Autodesk Inventor part; units mm, degrees
ref_plane "YZ Plane" through (0, 0, 0) normal (1, 0, 0) x (0, 1, 0)
ref_plane "XZ Plane" through (0, 0, 0) normal (0, 1, 0) x (-1, 0, 0)
ref_plane "XY Plane" through (0, 0, 0) normal (0, 0, 1) x (1, 0, 0)
sketch "Skizze1" plane through (0, 0, 0) normal (0, 1, 0) x (-1, 0, 0)
  circle A0 centre (0, 0) radius 45
  circle A1 centre (0, 0) radius 47.5
  dimension "d0" = 90
  dimension "d1" = 95
extrude "Extrusion1" add sketch "Skizze1" along normal blind 10
sketch "Skizze2" plane through (0, 0, 0) normal (0, -1, 0) x (1, 0, 0)
  circle A0 centre (0, 0) radius 41.5
  circle A1 centre (0, 0) radius 50
  dimension "d4" = 83
  dimension "d5" = 100
extrude "Extrusion2" add sketch "Skizze2" along normal blind 3
sketch "Skizze3" plane through (0, -3, 0) normal (0, -1, 0) x (1, 0, 0)
  circle A0 centre (0, 0) radius 41.5
  circle A1 centre (0, 0) radius 44
  dimension "d8" = 83
  dimension "d9" = 88
extrude "Extrusion3" add sketch "Skizze3" along normal blind 5
sketch "Skizze4" plane through (0, 0, 0) normal (0, 1, 0) x (1, 0, 0)
  line L0 (-86, 0) -> (65, 0) construction
  line L1 (-86, 15) -> (65, 15)
  line L2 (-86, -15) -> (65, -15)
  line L3 (-86, 15) -> (-86, -15)
  line L4 (65, -15) -> (65, 15)
  point P0 (0, 0)
  dimension "d12" = 15
  dimension "d13" = 15
extrude "Extrusion4" cut sketch "Skizze4" along normal up to surface (10 mm away)
sketch "Skizze5" plane through (0, 10, 0) normal (0, 1, 0) x (1, 0, 0)
  line L0 (0, 0) -> (0, 69) construction
  line L1 (-1.5, 0) -> (-1.5, 46.3972)
  line L2 (1.5, 0) -> (1.5, 46.3972)
  line L3 (-1.5, 0) -> (1.5, 0)
  line L4 (-1.5, 46.3972) -> (1.5, 46.3972)
  dimension "d16" = 1.5
extrude "Extrusion5" cut sketch "Skizze5" against normal up to surface (10 mm away)
properties part number "Teesiebhalter"
For this review, take the finished solid that the model builds, in its own axes (mm). A direction names the side the tool comes from. Give positions to 0.01 mm unless a question says otherwise; leave off trailing zeros. Loops run counter-clockwise (first coordinate to the right, second up) from the corner with the lowest first, then second, coordinate; pieces in that order, holes last.
Item 1: Take a section at D-D, the plane z = 36.5. State the section outline as (x, y) points.
Item 2: Take a section at C-C, the plane x = 0. State the section outline as (y, z) points, and give its area (3 significant figures).
Item 3: Take a section at B-B, the plane y = 2.75. State the section outline as (x, z) points (3 decimals), and give its area (3 significant figures).
Item 4: Insertion check: pin 1 (8 mm diameter, centred on y = -3.5, z = -12.5, fed in from -X); pin 2 (8 mm diameter, centred on x = 25.5, z = 28.5, fed in from +Y); pin 3 (10 mm diameter, centred on x = 7, y = 2, fed in from +Z); pin 4 (10 mm diameter, centred on y = 6, z = 4, fed in from -X). Each pin has a flat end and moves straight along its axis. Give the tip position at first contact, or say it passes through.
Item 5: Tool access review of faces 4 (the flat face through (-44, 5, 15)), 5 (the cylindrical face through (0.831, 4.93, 47.493)), 6 (the cylindrical face through (26.28, 4.93, -36.53)): name each direction out of +Z, -Z, +X, -X, +Y, -Y from which nothing blocks a thin tool from reaching the whole face with its end or side.
Item 6: Take a section at A-A, the plane z = 0. State the section outline as (x, y) points.
Item 7: Draft analysis for pull direction X (two halves, no side actions). For faces 1 (the flat face through (44, 5, -15)), 2 (the cylindrical face through (-0.831, 4.93, -47.493)), 3 (the cylindrical face through (0.775, 4.93, 44.993)), state which applies: +X half, -X half, draft (parallel to the pull), parting line (faces both ways), or undercut.
Item 8: For line 1 along Z through (x, y) = (0, -1.5); line 2 along Z through (x, y) = (0, -4.75); line 3 along Y through (x, z) = (-37, -27), list the stretches that pass through material, from the lowest coordinate up.
Calculated:
1. outline: (-34.17, -3) - (-24.57, -3) - (-24.57, -8) - (-19.75, -8) - (-19.75, 0) - (-26.32, 0) - (-26.32, 10) - (-30.4, 10) - (-30.4, 0) - (-34.17, 0) - close; (19.75, -8) - (24.57, -8) - (24.57, -3) - (34.17, -3) - (34.17, 0) - (30.4, 0) - (30.4, 10) - (26.32, 10) - (26.32, 0) - (19.75, 0) - close
2. outline: (-8, -44) - (-3, -44) - (-3, -50) - (0, -50) - (0, -47.5) - (10, -47.5) - (10, -46.4) - (0, -46.4) - (0, -41.5) - (-8, -41.5) - close; (-8, 41.5) - (0, 41.5) - (0, 45) - (10, 45) - (10, 47.5) - (0, 47.5) - (0, 50) - (-3, 50) - (-3, 44) - (-8, 44) - close
2. area: 112 mm2
3. outline: (-45.069, -15) arc R47.5 ccw to (45.069, -15) - (42.426, -15) arc R45 cw to (1.5, -44.975) - (1.5, -46.397) - (-1.5, -46.397) - (-1.5, -44.975) arc R45 cw to (-42.426, -15) - close; (-45.069, 15) - (-42.426, 15) arc R45 cw to (42.426, 15) - (45.069, 15) arc R47.5 ccw to start
3. area: 570 mm2
4. pin 1: stops at x = -49.27
4. pin 2: stops at y = 0
4. pin 3: stops at z = 49.94
4. pin 4: passes through
5. face 4: +X, -X, +Y
5. face 5: +Z, +Y
5. face 6: +Y
6. outline: (-50, -3) - (-44, -3) - (-44, -8) - (-41.5, -8) - (-41.5, 0) - (-50, 0) - close; (41.5, -8) - (44, -8) - (44, -3) - (50, -3) - (50, 0) - (41.5, 0) - close
7. face 1: draft
7. face 2: parting line
7. face 3: undercut
8. line 1: z = -50 to -41.5, 41.5 to 50
8. line 2: z = -44 to -41.5, 41.5 to 44
8. line 3: y = -3 to 10
